Could you check a few things on this model? Use its own coordinates, in mm. A direction names the side the tool comes from. Give positions to 0.01 mm unless a question says otherwise; leave off trailing zeros. Order: outer loops, then holes, each group sorted by start corner. A loop starts at its lowest first (then second) coordinate and runs counter-clockwise, first axis right, second up.
from build123d import *

# Parameters (mm, degrees)
EXTRUDE1_DEPTH                               = 200
FILLET1_R                                    = 0.5
CUT_EXTRUDE2_START                           = 200
SKETCH2_W                                    = 1.5
SKETCH2_H                                    = 54
CUT_EXTRUDE2_DEPTH                           = 112
CSK_FOR_M3_COUNTERSUNK_FLAT_HEAD_SCR_2_COUNT = 2
CSK_FOR_M3_COUNTERSUNK_FLAT_HEAD_SCR_2_PITCH = 192


with BuildPart() as part:
    # Sketch1 → Extrude1 (new body)
    with BuildSketch(Plane.XY):
        Polygon((0, 0), (13.5, 0), (13.5, 100), (12, 100), (12, 1.5), (0, 1.5), align=None)
    extrude(amount=EXTRUDE1_DEPTH)

    # Fillet1
    fillet1_edges = [part.edges().sort_by_distance(p)[0] for p in [
        (13.5, 0, 100),
    ]]
    fillet(fillet1_edges, radius=FILLET1_R)

    # Sketch2 → Cut-Extrude2 (cut)
    with BuildSketch(Plane.XY.offset(CUT_EXTRUDE2_START)):
        with Locations((12.75, 47.5)):
            Rectangle(SKETCH2_W, SKETCH2_H)
    extrude(amount=-CUT_EXTRUDE2_DEPTH, mode=Mode.SUBTRACT)

    # Sketch5 → CSK for M3 Countersunk Flat Head Screw1 (revolve, cut)
    with BuildSketch(Plane(origin=(6, 0, 196), x_dir=(0, 0, -1), z_dir=(1, 0, 0))):
        Polygon((0, 0), (0, 2.521463052), (1.7, 1.5), (1.7, 1.45), (3.15, 0), align=None)
    csk_for_m3_countersunk_flat_head_screw1 = revolve(axis=Axis((6, -6.35, 196), (0, 1, 0)), mode=Mode.SUBTRACT)

    # CSK for M3 Countersunk Flat Head Scr 2: CSK for M3 Countersunk Flat Head Screw1 ×2
    with Locations(*[(0, 0, -i * CSK_FOR_M3_COUNTERSUNK_FLAT_HEAD_SCR_2_PITCH) for i in range(1, CSK_FOR_M3_COUNTERSUNK_FLAT_HEAD_SCR_2_COUNT)]):
        add(csk_for_m3_countersunk_flat_head_screw1, mode=Mode.SUBTRACT)


solid = part.part
Item 1: Imagine slicing it at C-C on y = 29. List the corners of the cut face in (x, z) for me.
Findings:
outline: (12, 0) - (13.5, 0) - (13.5, 88) - (12, 88) - close
Item 2: Imagine slicing it at D-D on y = 89.5. List the corners of the cut face in (x, z) for me.
Findings:
outline: (12, 0) - (13.5, 0) - (13.5, 200) - (12, 200) - close
Item 3: For faces 1 (the flat face through (13.5, 50, 76)), 2 (the flat face through (6, 1.5, 99)), which set-ups out of +Z, -Z, +X, -X, +Y, -Y let a thin tool reach every point of the face, with its end or its side?
Findings:
face 1: +Z, -Z, +X, +Y, -Y
face 2: +Z, -Z, -X, +Y
Item 4: Please list where these lines run through material, in increasing order: line 1 along Y through (x, z) = (12.5, 158.5); line 2 along Y through (x, z) = (6.25, 128); line 3 along X through (y, z) = (1.55, 196).
Findings:
line 1: y = 0 to 20.5, 74.5 to 100
line 2: y = 0 to 1.5
line 3: x = 12 to 13.5
Item 5: For pin 1 (2 mm diameter, centred on x = 9, z = 132.5, fed in from +Y); pin 2 (5 mm diameter, centred on y = 19, z = 163, fed in from -X), each with a flat end and sliding along its axis, tell me the tip position at first contact or that it passes through.
Findings:
pin 1: stops at y = 1.5
pin 2: stops at x = 12
Item 6: Imagine slicing it at A-A on z = 180. List the corners of the cut face in (x, y) for me.
Findings:
outline: (0, 0) - (13, 0) arc R0.5 ccw to (13.5, 0.5) - (13.5, 20.5) - (12, 20.5) - (12, 1.5) - (0, 1.5) - close; (12, 74.5) - (13.5, 74.5) - (13.5, 100) - (12, 100) - close
Item 7: Imagine slicing it at B-B on z = 55. List the corners of the cut face in (x, y) for me, then the cut area to 3 significant figures.
Findings:
outline: (0, 0) - (13, 0) arc R0.5 ccw to (13.5, 0.5) - (13.5, 100) - (12, 100) - (12, 1.5) - (0, 1.5) - close
area: 168 mm2
